Could you check a few things on this model? Use its own coordinates, in mm. Give positions to 0.01 mm unless a question says otherwise; leave off trailing zeros. Loops run counter-clockwise (first coordinate to the right, second up) from the corner with the lowest first, then second, coordinate; pieces in that order, holes last. Notation, with made-up numbers: (3, 42.5) - (41, 42.5) arc R12 cw to (41, 55.5) - close; hole circle Ø8 at (-5.5, -13.75). An arc over 180 degrees is marked (long way). Answer in a Markdown table with one row per item. Add a question column.
```python
from build123d import *

# Parameters (mm, degrees)
SKETCH1_R           = 2
BOSS_EXTRUDE1_DEPTH = 0.5


with BuildPart() as part:
    # Sketch1 → Boss-Extrude1 (new body)
    with BuildSketch(Plane.XY):
        with BuildLine():
            Line((0, 5), (0, 80))
            ThreePointArc((0, 80), (-1.464466094, 83.535533906), (-5, 85))
            Line((-5, 85), (-12.03559932, 85))
            ThreePointArc((-12.03559932, 85), (-14.877749771, 84.587605583), (-17.485482826, 83.384436163))
            Line((-17.485482826, 83.384436163), (-110.449883506, 22.957575721))
            ThreePointArc((-110.449883506, 22.957575721), (-113.78916478, 19.342896624), (-115, 14.573139558))
            Line((-115, 14.573139558), (-115, 5))
            ThreePointArc((-115, 5), (-113.535533906, 1.464466094), (-110, 0))
            Line((-110, 0), (-5, 0))
            ThreePointArc((-5, 0), (-1.464466094, 1.464466094), (0, 5))
        make_face()
        with Locations((-105, 5)):
            Circle(SKETCH1_R, mode=Mode.SUBTRACT)
        with Locations((-25, 5)):
            Circle(SKETCH1_R, mode=Mode.SUBTRACT)
        with Locations((-5, 30)):
            Circle(SKETCH1_R, mode=Mode.SUBTRACT)
        with Locations((-5, 65)):
            Circle(SKETCH1_R, mode=Mode.SUBTRACT)
    extrude(amount=BOSS_EXTRUDE1_DEPTH)


solid = part.part
```
(1) We'd pull the mould along X, two halves only. Please class faces 1 (the flat face through (-46, 34, 0)), 2 (the cylindrical face through (-26.998, 5.088, 0.246)), 3 (the cylindrical face through (-113.57, 1.5, 0.25)): pulls with the +X half, pulls with the -X half, needs draft (parallel to the pull), parting line crosses it, or undercut.
(2) I want a section at A-A on x = -25. Please give me the cut outline in (y, z).
(3) Please list where these lines run through material, in increasing order: line 1 (Y direction, x = -5, z = 0.3); line 2 (X direction, y = 66.5, z = 0.2); line 3 (X direction, y = 29, z = 0.05).
(4) I want a section at B-B on z = 0.25. Please give me the cut outline in (x, y), then the cut area to 3 significant figures.
(5) I want a section at D-D on x = -53. Please give me the cut outline in (y, z), then the cut area to 4 significant figures.
(6) I want a section at C-C on y = 65. Please give me the cut outline in (x, z), then the cut area to 3 significant figures.
Reported:
| question | item | result |
|---|---|---|
| 1 | face 1 | needs draft |
| 1 | face 2 | undercut |
| 1 | face 3 | pulls with the -X half |
| 2 | outline | (0, 0) - (3, 0) - (3, 0.5) - (0, 0.5) - close; (7, 0) - (78.5, 0) - (78.5, 0.5) - (7, 0.5) - close |
| 3 | line 1 | 0 to 28, 32 to 63, 67 to 85 |
| 3 | line 2 | -43.46 to -6.32, -3.68 to 0 |
| 3 | line 3 | -101.15 to -6.73, -3.27 to 0 |
| 4 | outline | (-115, 5) arc R5 ccw to (-110, 0) - (-5, 0) arc R5 ccw to (0, 5) - (0, 80) arc R5 ccw to (-5, 85) - (-12.04, 85) arc R10 ccw to (-17.49, 83.38) - (-110.45, 22.96) arc R10 ccw to (-115, 14.57) - close; hole circle Ø4 at (-105, 5); hole circle Ø4 at (-25, 5); hole circle Ø4 at (-5, 30); hole circle Ø4 at (-5, 65) |
| 4 | area | 6,450 mm² |
| 5 | outline | (0, 0) - (60.3, 0) - (60.3, 0.5) - (0, 0.5) - close |
| 5 | area | 30.15 mm² |
| 6 | outline | (-45.77, 0) - (-7, 0) - (-7, 0.5) - (-45.77, 0.5) - close; (-3, 0) - (0, 0) - (0, 0.5) - (-3, 0.5) - close |
| 6 | area | 20.9 mm² |
